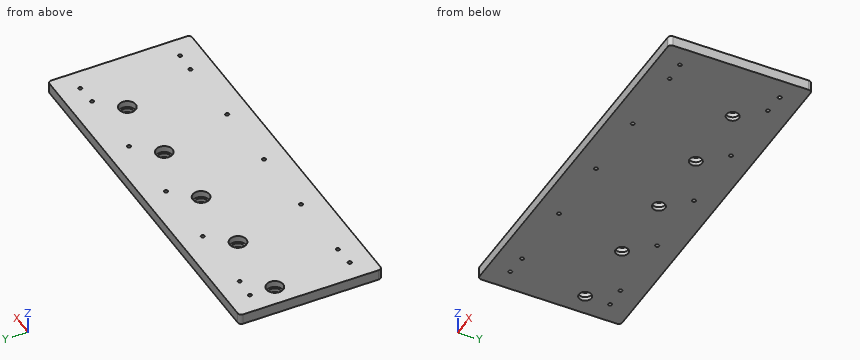
from build123d import *

# Parameters (mm, degrees)
SKETCH2_W               = 660.4
SKETCH2_H               = 254
BOSS_EXTRUDE1_DEPTH     = 19.05
F_1_4_CLEARANCE_HOLE1_D = 6.5278
FILLET1_R               = 6.35
F_1_4_CLEARANCE_HOLE2_D = 6.5278
SKETCH10_R              = 11.1125
CUT_EXTRUDE1_DEPTH      = 355.293582358
SKETCH12_R              = 14.859
CUT_EXTRUDE2_DEPTH      = 11.938


with BuildPart() as part:
    # Sketch2 → Boss-Extrude1 (new body)
    with BuildSketch(Plane.XY):
        Rectangle(SKETCH2_W, SKETCH2_H)
    extrude(amount=BOSS_EXTRUDE1_DEPTH)

    # 1/4 Clearance Hole1 (through all)
    with Locations(Plane.XY.offset(19.05)):
        with Locations((-254, -87.376), (-254, 87.376), (-127, 87.376), (0, 87.376), (127, 87.376), (254, 87.376), (-127, -87.376), (0, -87.376), (127, -87.376), (254, -87.376)):
            Hole(F_1_4_CLEARANCE_HOLE1_D / 2)

    # Fillet1
    fillet1_edges = [part.edges().sort_by_distance(p)[0] for p in [
        (330.2, -127, 9.525),
        (-330.2, -127, 9.525),
        (-330.2, 127, 9.525),
        (330.2, 127, 9.525),
    ]]
    fillet(fillet1_edges, radius=FILLET1_R)

    # 1/4 Clearance Hole2 (through all)
    with Locations(Plane.XY.offset(19.05)):
        with Locations((-292.1, 88.9), (292.1, -88.9), (-292.1, -88.9), (292.1, 88.9)):
            Hole(F_1_4_CLEARANCE_HOLE2_D / 2)

    # Sketch10 → Cut-Extrude1 (cut, through all)
    with BuildSketch(Plane(origin=(0, 0, 0), x_dir=(-1, 0, 0), z_dir=(0, 0, -1))):
        with Locations((-215.9, 44.45)):
            Circle(SKETCH10_R)
        with Locations((-88.9, 44.45)):
            Circle(SKETCH10_R)
        with Locations((38.1, 44.45)):
            Circle(SKETCH10_R)
        with Locations((165.1, 44.45)):
            Circle(SKETCH10_R)
        with Locations((292.1, 44.45)):
            Circle(SKETCH10_R)
    extrude(amount=-CUT_EXTRUDE1_DEPTH, mode=Mode.SUBTRACT)

    # Sketch12 → Cut-Extrude2 (cut)
    with BuildSketch(Plane.XY.offset(19.05)):
        with Locations((-292.1, 44.45)):
            Circle(SKETCH12_R)
        with Locations((-165.1, 44.45)):
            Circle(SKETCH12_R)
        with Locations((-38.1, 44.45)):
            Circle(SKETCH12_R)
        with Locations((88.9, 44.45)):
            Circle(SKETCH12_R)
        with Locations((215.9, 44.45)):
            Circle(SKETCH12_R)
    extrude(amount=-CUT_EXTRUDE2_DEPTH, mode=Mode.SUBTRACT)


solid = part.part
For this review, take the finished solid that the model builds, in its own axes (mm). Coordinates: 2 decimals unless noted, no trailing zeros. Order: outer loops, then holes, each group sorted by start corner. A loop starts at its lowest first (then second) coordinate and runs counter-clockwise, first axis right, second up. Notation, with made-up numbers: (76, 59.5) -> (106, 59.5) arc R3 ccw to (106, 64.5) -> close; hole circle Ø3 at (-12, 32). An arc over 180 degrees is marked (long way). Return JSON: item names as keys, results as strings.
1. For pin 1 Ø24 at (x, y) = (215.9, 44.45) entering from +Z, flat-tipped, find the tip position at first contact; note if it passes through.
Answer block:
{"pin 1": "z = 7.11"}
2. We need section A-A on x = -165.1. Write out the cut boundary in (y, z), and give its area (3 significant figures).
Answer block:
{"outline": "(-127, 0) -> (33.34, 0) -> (33.34, 7.11) -> (29.59, 7.11) -> (29.59, 19.05) -> (-127, 19.05) -> close; (55.56, 0) -> (127, 0) -> (127, 19.05) -> (59.31, 19.05) -> (59.31, 7.11) -> (55.56, 7.11) -> close", "area": "4,330 mm²"}
3. We need section B-B on z = 14.75. State how many separate pieces and enclosed holes the cut face has, and give its area (3 significant figures).
Answer block:
{"separate pieces": "1", "enclosed holes": "19", "area": "164,000 mm²"}
4. For line 1 (Y direction, x = -127, z = 4.75); line 2 (Y direction, x = -292.1, z = 9.5); line 3 (Y direction, x = 88.9, z = 16.5), list the stretches that pass through material, from the lowest coordinate up. Write a range as from..to.
Answer block:
{"line 1": "-127..-90.64, -84.11..84.11, 90.64..127", "line 2": "-127..-92.16, -85.64..29.59, 59.31..85.64, 92.16..127", "line 3": "-127..29.59, 59.31..127"}
